Verification items for the finished model (mm, model axes). A direction names the side the tool comes from. Give positions to 0.01 mm unless a question says otherwise; leave off trailing zeros. Loops run counter-clockwise (first coordinate to the right, second up) from the corner with the lowest first, then second, coordinate; pieces in that order, holes last. Notation, with made-up numbers: (53, 68) -> (83, 68) arc R12 ccw to (83, 91) -> close; hole circle Ø11 at (38.25, 58.5). An arc over 180 degrees is marked (long way). Answer in a Markdown table with one row per item. Add a question column.
Q1. Section check A-A on x = 0. Enter the section's corners in (y, z), and give its area (3 significant figures).
Q2. Section check D-D on x = -8.75. Enter the section's corners in (y, z) (3 decimals).
Q3. Gauge pin test, flat ends, axial feed: P1, Ø16.5, axis at x = 0, y = 0, coming from the +Z side; P2, Ø1, axis at x = -2, z = 5, coming from the -Y side; P3, Ø2, axis at x = -5, z = 7, coming from the +Y side; P4, Ø3, axis at y = 9.525, z = 5.207, coming from the +X side. Record the tip position at first contact, or that the pin passes through.
Q4. Section check C-C on y = 5.5. Enter the section's corners in (x, z).
Q5. Section check B-B on z = 1.5. Enter the section's corners in (x, y), and give its area (3 significant figures).
Q6. Set-up check for faces 1 (the face through (-8.49, 11.49, 5.46)), 2 (the face through (8.49, -11.49, 5.46)), 3 (the face through (1.265, 11.237, 5.134)): record each of +Z, -Z, +X, -X, +Y, -Y from which the full face is reachable in a straight line by a thin tool's end or side.
Q7. Release check for a two-part mould opening along Z. For faces 4 (the face through (10.986, -0.073, 5.134)), 5 (the face through (-8.49, -8.19, 6.67)), 6 (the face through (-7, -4, 10.414)) record: pulls with the +Z half, pulls with the -Z half, needs draft (parallel to the pull), parting line crosses it, or undercut.
Q8. Material ranges on probe 1 along Y at (x, z) = (2, 10); probe 2 along Y at (x, z) = (-13, 6.25); probe 3 along Y at (x, z) = (13, 8.25), recorded low to high.
Autodesk Inventor part; units mm, degrees
ref_plane "YZ Plane" through (0, 0, 0) normal (1, 0, 0) x (0, 1, 0)
ref_plane "XZ Plane" through (0, 0, 0) normal (0, 1, 0) x (-1, 0, 0)
ref_plane "XY Plane" through (0, 0, 0) normal (0, 0, 1) x (1, 0, 0)
sketch "Sketch1" plane through (0, 0, 0) normal (0, 0, 1) x (1, 0, 0)
  circle A0 centre (0, 0) radius 7.1437
  circle A1 centre (0, 0) radius 20.32
  dimension "d0" = 14.2875
  dimension "d1" = 40.64
extrude "Extrusion1" add sketch "Sketch1" along normal blind 10.414
thread "Thread1"
sketch "Sketch2" plane through (0, 0, 10.414) normal (0, 0, 1) x (1, 0, 0)
  point P0 (0, 0)
  point P1 (0, 14.2875)
  dimension "d6" = 14.2875
hole "Hole1" at (0, 14.2875, 10.414) direction (0, 0, -1) diameter 6.604 depth 12.2936 tip angle 118
pattern_circular "Circular Pattern1" count 4 over 360 about axis through (0, 0, 0) along (0, 0, 1) of "Hole1"
sketch "Sketch3" plane through (0, 0, 10.414) normal (0, 0, 1) x (1, 0, 0)
  line L0 (-14.2875, -29.4711) -> (14.2875, -29.4711)
  line L1 (14.2875, -29.4711) -> (14.2875, 27.3802)
  line L2 (14.2875, 27.3802) -> (-14.2875, 27.3802)
  line L3 (-14.2875, 27.3802) -> (-14.2875, -29.4711)
  line L4 (-49.0321, -62.4929) -> (63.3318, -62.4929)
  line L5 (63.3318, -62.4929) -> (63.3318, 57.2179)
  line L6 (63.3318, 57.2179) -> (-49.0321, 57.2179)
  line L7 (-49.0321, 57.2179) -> (-49.0321, -62.4929)
  point P0 (0, 0)
  dimension "d17" = 28.575
  dimension "d18" = 14.2875
extrude "Extrusion2" cut sketch "Sketch3" against normal blind 10.414
sketch "Sketch4" plane through (14.2875, 3.302, 10.414) normal (1, 0, 0) x (0, 0, -1)
  line L0 (0, -6.604) -> (10.414, -6.604)
  line L1 (10.414, 0) -> (10.414, -6.604)
  line L2 (10.414, 0) -> (0, 0)
  line L3 (0, -6.604) -> (0, 0)
  line L4 (0, -3.302) -> (10.414, -3.302)
  point P0 (5.207, 6.223)
  point P1 (5.207, -3.302)
  point P2 (5.207, -12.827)
  dimension "d21" = 9.525
  dimension "d22" = 9.525
hole "Hole2" at (14.2875, 9.525, 5.207) at (14.2875, -9.525, 5.207) direction (-1, 0, 0) diameter 3.9624 depth 11.43 tip angle 118
mirror "Mirror1" about plane through (0, 0, 0) normal (1, 0, 0) of "Hole2"
Taken from the geometry:
| question | item | result |
|---|---|---|
| 1 | outline | (-20.32, 0) -> (-17.59, 0) -> (-17.59, 10.41) -> (-20.32, 10.41) -> close; (-10.99, 0) -> (-7.14, 0) -> (-7.14, 10.41) -> (-10.99, 10.41) -> close; (7.14, 0) -> (10.99, 0) -> (10.99, 10.41) -> (7.14, 10.41) -> close; (17.59, 0) -> (20.32, 0) -> (20.32, 10.41) -> (17.59, 10.41) -> close |
| 1 | area | 137 mm² |
| 2 | outline | (-18.34, 0) -> (18.34, 0) -> (18.34, 10.414) -> (-18.34, 10.414) -> close; hole circle Ø3.962 at (-9.525, 5.207); hole circle Ø3.962 at (9.525, 5.207) |
| 3 | P1 | stops at z = 10.41 |
| 3 | P2 | stops at y = -20.26 |
| 3 | P3 | stops at y = 19.92 |
| 3 | P4 | stops at x = 2.57 |
| 4 | outline | (-14.29, 0) -> (-4.56, 0) -> (-4.56, 10.41) -> (-14.29, 10.41) -> close; (4.56, 0) -> (14.29, 0) -> (14.29, 10.41) -> (4.56, 10.41) -> close |
| 5 | outline | (-14.29, -14.45) arc R20.32 ccw to (14.29, -14.45) -> (14.29, -3.3) arc R3.3 cw to (14.29, 3.3) -> (14.29, 14.45) arc R20.32 ccw to (-14.29, 14.45) -> (-14.29, 3.3) arc R3.3 cw to (-14.29, -3.3) -> close; hole circle Ø14.29 at (0, 0); hole circle Ø6.6 at (0, -14.29); hole circle Ø6.6 at (0, 14.29) |
| 5 | area | 794 mm² |
| 6 | face 1 | -X |
| 6 | face 2 | +X |
| 6 | face 3 | +Z, -Z |
| 7 | face 4 | needs draft |
| 7 | face 5 | undercut |
| 7 | face 6 | pulls with the +Z half |
| 8 | probe 1 | y = -20.22 to -16.91, -11.66 to -6.86, 6.86 to 11.66, 16.91 to 20.22 |
| 8 | probe 2 | y = -15.62 to -11.21, -7.84 to -3.04, 3.04 to 7.84, 11.21 to 15.62 |
| 8 | probe 3 | y = -15.62 to -3.04, 3.04 to 15.62 |
